from build123d import *

# Parameters (mm, degrees)
BASE_FLANGE1_DEPTH   = 3.175
EDGE_FLANGE1_DEPTH   = 15
EDGE_FLANGE2_DEPTH   = 15
BOSS_EXTRUDE1_DEPTH  = 3.175
M5_CLEARANCE_HOLE1_D = 5.5
FILLET1_R            = 3.175
M8_CLEARANCE_HOLE1_D = 9


# Sheet-metal steps are written as plain solids
with BuildPart() as part:
    # Sketch2 → Base-Flange1 (new body)
    with BuildSketch(Plane.XY):
        Polygon((-136.862074611, 27.127820722), (-140.037074611, 21.628559408), (-153.027455668, 29.128559408), (-149.852455668, 34.627820722), (-139.057455668, 53.32530919), (-126.067074611, 45.82530919), align=None)
    extrude(amount=BASE_FLANGE1_DEPTH)

    # Edge-Flange1 section (across the edge) → Edge-Flange1 (add)
    with BuildSketch(Plane(origin=(-138.263705668, 54.700124518, 0), x_dir=(-0.49999999999999706, -0.8660254037844405, -3.491481338843133e-15), z_dir=(0.8660254037844405, -0.49999999999999706, 0))):
        with BuildLine():
            Line((-3.175, 1.5875), (-3.175, 27.899995))
            Line((-3.175, 27.899995), (0, 27.899995))
            Line((0, 27.899995), (0, 1.5875))
            ThreePointArc((0, 1.5875), (0.464967985, 0.464967985), (1.5875, 0))
            Line((1.5875, 0), (1.5875, -3.175))
            ThreePointArc((1.5875, -3.175), (-1.780096045, -1.780096045), (-3.175, 1.5875))
        make_face()
    extrude(amount=EDGE_FLANGE1_DEPTH)

    # Edge-Flange2 section (across the edge) → Edge-Flange2 (add)
    with BuildSketch(Plane(origin=(-123.685824611, 49.949755175, -29.487495), x_dir=(0, 0, 1), z_dir=(-0.8660254037844397, 0.4999999999999983, 0))):
        with BuildLine():
            Line((-3.175, 1.5875), (-3.175, 6.35))
            Line((-3.175, 6.35), (0, 6.35))
            Line((0, 6.35), (0, 1.5875))
            ThreePointArc((0, 1.5875), (0.464967985, 0.464967985), (1.5875, 0))
            Line((1.5875, 0), (1.5875, -3.175))
            ThreePointArc((1.5875, -3.175), (-1.780096045, -1.780096045), (-3.175, 1.5875))
        make_face()
    extrude(amount=EDGE_FLANGE2_DEPTH)

    # Sketch15 → Boss-Extrude1 (add)
    with BuildSketch(Plane(origin=(0, 0, -32.662495), x_dir=(-1, 0, 0), z_dir=(0, 0, -1))):
        Polygon((133.501205668, 62.949016489), (120.510824611, 55.449016489), (115.748324611, 63.69790846), (115.748324611, 78.93790846), (130.748324611, 78.93790846), (130.748324611, 67.717146347), align=None)
    extrude(amount=-BOSS_EXTRUDE1_DEPTH)

    # M5 Clearance Hole1 (through all)
    with Locations(Plane.XY.offset(3.175)):
        with Locations((-143.35726514, 30.877820722)):
            Hole(M5_CLEARANCE_HOLE1_D / 2)

    # Fillet1
    fillet1_edges = [part.edges().sort_by_distance(p)[0] for p in [
        (-140.037074611, 21.628559408, 1.5875),
        (-153.027455668, 29.128559408, 1.5875),
        (-130.748324611, 67.717146347, -31.074995),
        (-115.748324611, 63.69790846, -31.074995),
        (-115.748324611, 78.93790846, -31.074995),
        (-130.748324611, 78.93790846, -31.074995),
    ]]
    fillet(fillet1_edges, radius=FILLET1_R)

    # M8 Clearance Hole1 (through all)
    with Locations(Plane.XY.offset(-29.487495)):
        with Locations((-123.248324611, 69.41100346)):
            Hole(M8_CLEARANCE_HOLE1_D / 2)


solid = part.part
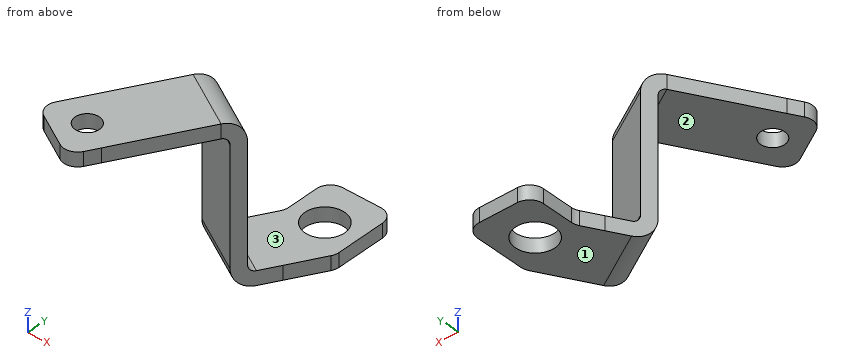
Work out the finished part from the listing and answer in its coordinate system (mm). Face numbers are marked on the shaded views. A direction names the side the tool comes from. Round coordinates to 2 decimals unless told otherwise and drop trailing zeros. Write each loop counter-clockwise with the first axis right and the second up, starting at its lowest first coordinate (ties: lowest second). Pieces come first, ordered by that corner, then holes.
1) A cutting plane is placed at B-B (y = 33). Give the vertices of the cut face in (x, z) (3 decimals), plus the area to 3 significant figures.
2) A cutting plane is placed at C-C (z = -15). Give the vertices of the cut face in (x, y).
3) A cutting plane is placed at D-D (y = 42.5). Give the vertices of the cut face in (x, z) (3 decimals).
4) Given pin 1 Ø10 at (x, z) = (-121, -7) entering from -Y; pin 2 Ø1.5 at (y, z) = (45.5, -21) entering from +X; pin 3 Ø3 at (x, y) = (-123.5, 49.5) entering from -Z; pin 4 Ø7 at (x, y) = (-143.36, 30.88) entering from -Z, each flat-ended and moving along its own axis, determine where each tip first touches the part or whether it passes through.
5) A tool of negligible diameter and unlimited length cuts with its end or side. For the marked faces 1, 2 and 3, from which of +Z, -Z, +X, -X, +Y, -Y can it reach the whole face along a straight path? Write none if from no direction.
6) Straight lines are drawn through the part: line 1 (Z direction, x = -143, y = 40.5) (3 decimals); line 2 (Z direction, x = -133, y = 61.5); line 3 (Y direction, x = -132, z = -1). For each, find the intervals that lie inside material, in ascending order.
7) A cutting plane is placed at A-A (x = -122). Give the vertices of the cut face in (y, z).
Completed:
1. outline: (-150.792, 0) - (-145.106, 0) - (-145.106, 3.175) - (-150.792, 3.175) - close; (-141.608, 0) - (-133.472, 0) - (-133.472, 3.175) - (-141.608, 3.175) - close
1. area: 43.9 mm2
2. outline: (-138.26, 54.7) - (-125.27, 47.2) - (-123.69, 49.95) - (-136.68, 57.45) - close
3. outline: (-145.307, 0) - (-127.987, 0) - (-127.987, 3.175) - (-145.307, 3.175) - close
4. pin 1: stops at y = 47.2
4. pin 2: passes through
4. pin 3: stops at z = -32.64
4. pin 4: stops at z = 0
5. face 1: -Z, +X, -X, +Y, -Y
5. face 2: -Z, -X, -Y
5. face 3: +Z, +X, +Y
6. line 1: z = 0 to 3.175
6. line 2: z = -32.66 to -29.49
6. line 3: y = 50.95 to 54.71
7. outline: (52.87, -32.66) - (65.09, -32.66) - (65.09, -29.49) - (52.87, -29.49) - close; (73.73, -32.66) - (78.94, -32.66) - (78.94, -29.49) - (73.73, -29.49) - close
